CAD build for the part. Positions are in the model's coordinates, mm. Round coordinates to 2 decimals unless told otherwise and drop trailing zeros. Write each loop counter-clockwise with the first axis right and the second up, starting at its lowest first coordinate (ties: lowest second). Pieces come first, ordered by that corner, then holes. Notation, with made-up numbers: (58.25, 42.5) -> (101.25, 42.5) arc R23 cw to (101.25, 72.5) -> close; hole circle Ø11 at (-37.75, 73). An arc over 180 degrees is marked (long way). Put each result on its own line as item: value. Start each with the question number.
1. Flat gauge pins, fed straight in: P1, Ø5, axis at y = 122.5, z = -4.5, coming from the -X side; P2, Ø2.5, axis at x = 1.5, z = -4.5, coming from the -Y side; P3, Ø2.5, axis at y = 123.5, z = -3.5, coming from the +X side; P4, Ø6.5, axis at y = 21, z = -3, coming from the +X side. Where does each tip first touch, or does it go through?
2. Saw through at B-B on x = 7.2. List the corners of the cut face in (y, z).
3. Drill centre lines: line 1 (Y direction, x = 7.2, z = -6); line 2 (Y direction, x = 100.5, z = -0.5); line 3 (Z direction, x = 103.15, y = 18.5). Where is each one in solid material? Low to high. Write a range as from..to.
4. Saw through at D-D on x = 40. List the corners of the cut face in (y, z).
5. Saw through at A-A on y = 128.5. List the corners of the cut face in (x, z), and give its area (3 significant figures).
6. Saw through at C-C on y = 89. List the corners of the cut face in (x, z).
from build123d import *

# Parameters (mm, degrees)
SKETCH1_W           = 113
SKETCH1_H           = 175.618176042
BOSS_EXTRUDE1_DEPTH = 0.8
SKETCH2_R           = 4
SKETCH2_R_2         = 2
BOSS_EXTRUDE2_DEPTH = 11
CUT_EXTRUDE1_DEPTH  = 3.5
SKETCH4_W           = 5
SKETCH4_H           = 8
BOSS_EXTRUDE3_DEPTH = 8
SKETCH5_R           = 1.75
CUT_EXTRUDE2_DEPTH  = 105
CUT_EXTRUDE3_DEPTH  = 2.5


with BuildPart() as part:
    # Sketch1 → Boss-Extrude1 (new body)
    with BuildSketch(Plane.XY):
        with Locations((52.5, 73.5)):
            Rectangle(SKETCH1_W, SKETCH1_H)
    extrude(amount=BOSS_EXTRUDE1_DEPTH)

    # Sketch2 → Boss-Extrude2 (add)
    with BuildSketch(Plane(origin=(0, 0, 0), x_dir=(-1, 0, 0), z_dir=(0, 0, -1))):
        with Locations((-7.2, 120.15)):
            Circle(SKETCH2_R)
        with Locations((-7.2, 120.15)):
            Circle(SKETCH2_R_2, mode=Mode.SUBTRACT)
        with Locations((-7.2, 26.85)):
            Circle(SKETCH2_R)
        with Locations((-7.2, 26.85)):
            Circle(SKETCH2_R_2, mode=Mode.SUBTRACT)
        with Locations((-101, 26.85)):
            Circle(SKETCH2_R)
        with Locations((-101, 26.85)):
            Circle(SKETCH2_R_2, mode=Mode.SUBTRACT)
        with Locations((-101, 120.15)):
            Circle(SKETCH2_R)
        with Locations((-101, 120.15)):
            Circle(SKETCH2_R_2, mode=Mode.SUBTRACT)
    extrude(amount=BOSS_EXTRUDE2_DEPTH)

    # Sketch3 → Cut-Extrude1 (cut)
    with BuildSketch(Plane(origin=(0, 0, 0), x_dir=(-1, 0, 0), z_dir=(0, 0, -1))):
        Polygon((-5.467949192, 123.15), (-8.932050808, 123.15), (-10.664101615, 120.15), (-8.932050808, 117.15), (-5.467949192, 117.15), (-3.735898385, 120.15), align=None)
        with BuildLine():
            Line((-10.664101615, 120.15), (-8.932050808, 123.15))
            Line((-8.932050808, 123.15), (-9.845751311, 123.15))
            ThreePointArc((-9.845751311, 123.15), (-11.2, 120.15), (-9.845751311, 117.15))
            Line((-9.845751311, 117.15), (-8.932050808, 117.15))
            Line((-8.932050808, 117.15), (-10.664101615, 120.15))
        make_face()
        Polygon((-102.732050808, 117.15), (-99.267949192, 117.15), (-97.535898385, 120.15), (-99.267949192, 123.15), (-102.732050808, 123.15), (-104.464101615, 120.15), align=None)
        with BuildLine():
            Line((-98.354248689, 123.15), (-99.267949192, 123.15))
            Line((-99.267949192, 123.15), (-97.535898385, 120.15))
            Line((-97.535898385, 120.15), (-99.267949192, 117.15))
            Line((-99.267949192, 117.15), (-98.354248689, 117.15))
            ThreePointArc((-98.354248689, 117.15), (-97.354248689, 118.504248689), (-97, 120.15))
            ThreePointArc((-97, 120.15), (-97.354248689, 121.795751311), (-98.354248689, 123.15))
        make_face()
        with BuildLine():
            Line((-99.267949192, 29.85), (-97.535898385, 26.85))
            Line((-97.535898385, 26.85), (-99.267949192, 23.85))
            Line((-99.267949192, 23.85), (-98.354248689, 23.85))
            ThreePointArc((-98.354248689, 23.85), (-97.354248689, 25.204248689), (-97, 26.85))
            ThreePointArc((-97, 26.85), (-97.354248689, 28.495751311), (-98.354248689, 29.85))
            Line((-98.354248689, 29.85), (-99.267949192, 29.85))
        make_face()
        Polygon((-102.732050808, 23.85), (-99.267949192, 23.85), (-97.535898385, 26.85), (-99.267949192, 29.85), (-102.732050808, 29.85), (-104.464101615, 26.85), align=None)
        Polygon((-5.467949192, 23.85), (-8.932050808, 23.85), (-10.664101615, 26.85), (-8.932050808, 29.85), (-5.467949192, 29.85), (-3.735898385, 26.85), align=None)
        with BuildLine():
            Line((-10.664101615, 26.85), (-8.932050808, 29.85))
            Line((-8.932050808, 29.85), (-9.845751311, 29.85))
            ThreePointArc((-9.845751311, 29.85), (-11.2, 26.85), (-9.845751311, 23.85))
            Line((-9.845751311, 23.85), (-8.932050808, 23.85))
            Line((-8.932050808, 23.85), (-10.664101615, 26.85))
        make_face()
    extrude(amount=CUT_EXTRUDE1_DEPTH, mode=Mode.SUBTRACT)

    # Sketch4 → Boss-Extrude3 (add)
    with BuildSketch(Plane(origin=(0, 0, 0), x_dir=(-1, 0, 0), z_dir=(0, 0, -1))):
        with Locations((-102.5, 18.5)):
            Rectangle(SKETCH4_W, SKETCH4_H)
        with BuildLine():
            Line((-105, 26.85), (-105, 22.5))
            Line((-105, 22.5), (-100, 22.5))
            Line((-100, 22.5), (-100, 22.977016654))
            ThreePointArc((-100, 22.977016654), (-103.449489743, 23.68772234), (-105, 26.85))
        make_face()
        with BuildLine():
            Line((-105, 124.5), (-105, 120.15))
            ThreePointArc((-105, 120.15), (-103.449489743, 123.31227766), (-100, 124.022983346))
            Line((-100, 124.022983346), (-100, 124.5))
            Line((-100, 124.5), (-105, 124.5))
        make_face()
        with Locations((-102.5, 128.5)):
            Rectangle(SKETCH4_W, SKETCH4_H)
        with BuildLine():
            Line((-3.2, 120.15), (-3.2, 124.5))
            Line((-3.2, 124.5), (-5, 124.5))
            Line((-5, 124.5), (-5, 123.490658618))
            ThreePointArc((-5, 123.490658618), (-3.678636628, 122.047366596), (-3.2, 120.15))
        make_face()
        with Locations((-2.5, 128.5)):
            Rectangle(SKETCH4_W, SKETCH4_H)
        Polygon((-5, 14.5), (0, 14.5), (0, 22.5), (-3.2, 22.5), (-5, 22.5), align=None)
        with BuildLine():
            Line((-5, 23.509341382), (-5, 22.5))
            Line((-5, 22.5), (-3.2, 22.5))
            Line((-3.2, 22.5), (-3.2, 26.85))
            ThreePointArc((-3.2, 26.85), (-3.678636628, 24.952633404), (-5, 23.509341382))
        make_face()
    extrude(amount=BOSS_EXTRUDE3_DEPTH)

    # Sketch5 → Cut-Extrude2 (cut)
    with BuildSketch(Plane.ZY.offset(-105)):
        with Locations((-3.896353455, 128.5)):
            Circle(SKETCH5_R)
        with Locations((-3.896353455, 18.5)):
            Circle(SKETCH5_R)
    extrude(amount=CUT_EXTRUDE2_DEPTH, mode=Mode.SUBTRACT)

    # Sketch6 → Cut-Extrude3 (cut)
    with BuildSketch(Plane.ZY.offset(-100)):
        Polygon((-3.896353455, 21.964101615), (-6.896353455, 20.232050808), (-6.896353455, 16.767949192), (-3.896353455, 15.035898385), (-0.896353455, 16.767949192), (-0.896353455, 20.232050808), align=None)
        Polygon((-0.896353455, 130.232050808), (-0.896353455, 126.767949192), (-3.896353455, 125.035898385), (-6.896353455, 126.767949192), (-6.896353455, 130.232050808), (-3.896353455, 131.964101615), align=None)
    cut_extrude3 = extrude(amount=-CUT_EXTRUDE3_DEPTH, mode=Mode.SUBTRACT)

    # Mirror1: Cut-Extrude3 across plane
    add(cut_extrude3.mirror(Plane.ZY.offset(-52.5)), mode=Mode.SUBTRACT)


solid = part.part
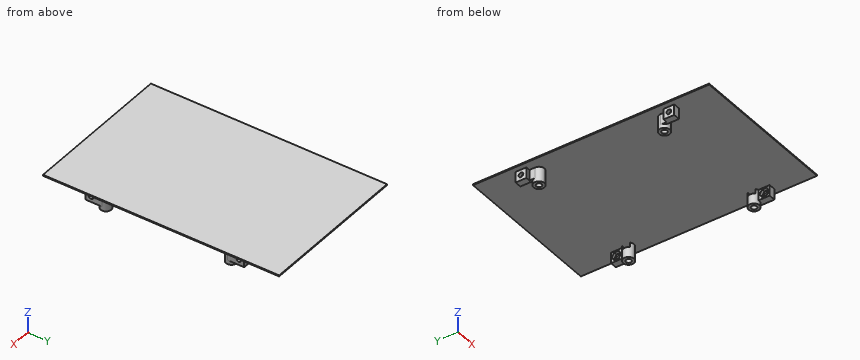
Return value:
1. P1: stops at x = 0
1. P2: stops at y = 14.5
1. P3: stops at x = 105
1. P4: stops at x = 109
2. outline: (-14.31, 0) -> (22.85, 0) -> (22.85, -11) -> (24.85, -11) -> (24.85, -3.5) -> (23.85, -3.5) -> (23.85, 0) -> (29.85, 0) -> (29.85, -3.5) -> (28.85, -3.5) -> (28.85, -11) -> (30.85, -11) -> (30.85, 0) -> (116.15, 0) -> (116.15, -11) -> (118.15, -11) -> (118.15, -3.5) -> (117.15, -3.5) -> (117.15, 0) -> (123.15, 0) -> (123.15, -3.5) -> (122.15, -3.5) -> (122.15, -11) -> (124.15, -11) -> (124.15, 0) -> (161.31, 0) -> (161.31, 0.8) -> (-14.31, 0.8) -> close
3. line 1: y = 22.85..24.85, 28.85..30.85, 116.15..118.15, 122.15..124.15
3. line 2: y = 14.5..23.85, 29.85..30.82, 116.18..117.15, 123.15..132.5
3. line 3: z = -8..-5.65, -2.15..0.8
4. outline: (-14.31, 0) -> (161.31, 0) -> (161.31, 0.8) -> (-14.31, 0.8) -> close
5. outline: (-4, 0) -> (0, 0) -> (0, -2.15) -> (2.5, -2.15) -> (2.5, -0.9) -> (5, -0.9) -> (5, 0) -> (100, 0) -> (100, -0.9) -> (102.5, -0.9) -> (102.5, -2.15) -> (105, -2.15) -> (105, 0) -> (109, 0) -> (109, 0.8) -> (-4, 0.8) -> close; (0, -8) -> (5, -8) -> (5, -6.9) -> (2.5, -6.9) -> (2.5, -5.65) -> (0, -5.65) -> close; (100, -8) -> (105, -8) -> (105, -5.65) -> (102.5, -5.65) -> (102.5, -6.9) -> (100, -6.9) -> close
5. area: 123 mm^2
6. outline: (-4, 0) -> (109, 0) -> (109, 0.8) -> (-4, 0.8) -> close
